Read the model definition and answer for the solid it produces. Units are mm, in the model's axes. A direction names the side the tool comes from. Give positions to 0.01 mm unless a question says otherwise; leave off trailing zeros. Loops run counter-clockwise (first coordinate to the right, second up) from the corner with the lowest first, then second, coordinate; pieces in that order, holes last. Notation, with made-up numbers: (57, 51.5) - (115, 51.5) arc R18 cw to (115, 69.5) - close; hole circle Ø9 at (-9, 38). An arc over 180 degrees is marked (long way). Write item = value, one per line.
```python
from build123d import *

# Parameters (mm, degrees)
F0_R      = 9.525
F1_DEPTH  = 15.8115
F2_R      = 11.1125
F3_DEPTH  = 7.112
F4_R      = 11.1125
F5_DEPTH  = 7.112
F6_T      = 3.175
F7_R      = 3.175
F8_DEPTH  = 3.175
F10_R     = 11.1125
F11_DEPTH = 1.5875


# Not quite as in the source:
# - a shell that OpenCascade refuses in one call is made with other operations: the cavity is built on its own and cut out


with BuildPart() as f1:
    # F0 (on Top) → F1 (new body)
    with BuildSketch(Plane.XY):
        with BuildLine():
            Line((-14.2875, 369.1638474552), (-14.2875, 0))
            ThreePointArc((-14.2875, 0), (-13.1999288208, -5.4675895399), (-10.1027881362, -10.1027881362))
            Line((-10.1027881362, -10.1027881362), (23.8125, -44.0180762724))
            Line((23.8125, -44.0180762724), (74.6125, -44.0180762724))
            Line((74.6125, -44.0180762724), (74.6125, 413.1819237276))
            Line((74.6125, 413.1819237276), (23.8125, 413.1819237276))
            Line((23.8125, 413.1819237276), (-10.1027881362, 379.2666355914))
            ThreePointArc((-10.1027881362, 379.2666355914), (-13.1999288208, 374.6314369951), (-14.2875, 369.1638474552))
        make_face()
        Circle(F0_R, mode=Mode.SUBTRACT)
        with Locations((0, 369.1638474552)):
            Circle(F0_R, mode=Mode.SUBTRACT)
    extrude(amount=F1_DEPTH)

    # F2 (on face) → F3 (cut)
    with BuildSketch(Plane.XY.offset(15.8115)):
        with Locations((0, 369.1638474552)):
            Circle(F2_R)
        Circle(F2_R)
    extrude(amount=-F3_DEPTH, mode=Mode.SUBTRACT)

    # F4 (on face) → F5 (cut)
    with BuildSketch(Plane(origin=(0, 0, 0), x_dir=(1, 0, 0), z_dir=(0, 0, -1))):
        Circle(F4_R)
        with Locations((0, -369.1638474552)):
            Circle(F4_R)
    extrude(amount=-F5_DEPTH, mode=Mode.SUBTRACT)

    # F6: shell of thickness 3.175, made by hand


with BuildPart() as f6_core1:
    # F6_t2: copy of F1
    add(f1.part)

    # the walls: a layer under each face that stays
    f6_faces = [f6_core1.faces().sort_by_distance(p)[0] for p in [
        (-13.1999288208, 374.6314369951, 7.90575),
        (6.8548559319, 396.2242796595, 7.90575),
        (-14.2875, 184.5819237276, 7.90575),
        (30.1625, 184.5819237276, 15.8115),
        (49.2125, 413.1819237276, 7.90575),
        (-13.1999288208, -5.4675895399, 7.90575),
        (74.6125, 184.5819237276, 7.90575),
        (6.8548559319, -27.0604322043, 7.90575),
        (49.2125, -44.0180762724, 7.90575),
        (-11.1125, 0, 3.556),
        (-11.1125, 369.1638474552, 3.556),
        (-11.1125, 0, 12.2555),
        (-11.1125, 369.1638474552, 12.2555),
        (-7.4083333333, 7.4083333333, 7.112),
        (-7.4083333333, 376.5721807885, 7.112),
        (-7.4083333333, -7.4083333333, 8.6995),
        (-7.4083333333, 361.7555141219, 8.6995),
        (-9.525, 0, 7.90575),
        (-9.525, 369.1638474552, 7.90575),
    ]]
    thicken(f6_faces, amount=-F6_T, mode=Mode.SUBTRACT)

    # F6_s3 → F6_t4 (revolve, cut)
    with BuildSketch(Plane.XZ):
        Polygon((11.08075, 7.08025), (14.2875, 7.112), (14.2875, 10.287), (11.1125, 10.287), align=None)
    revolve(axis=Axis((0, 0, 7.112), (0, 0, -1)), mode=Mode.SUBTRACT)

    # F6_s5 → F6_t6 (revolve, cut)
    with BuildSketch(Plane.XZ.offset(-369.1638474552)):
        Polygon((11.08075, 7.08025), (14.2875, 7.112), (14.2875, 10.287), (11.1125, 10.287), align=None)
    revolve(axis=Axis((0, 369.1638474552, 7.112), (0, 0, -1)), mode=Mode.SUBTRACT)

    # F6_s7 → F6_t8 (revolve, cut)
    with BuildSketch(Plane.XZ):
        Polygon((11.08075, 8.73125), (14.2875, 8.6995), (14.2875, 5.5245), (11.1125, 5.5245), align=None)
    revolve(axis=Axis((0, 0, 8.6995), (0, 0, 1)), mode=Mode.SUBTRACT)

    # F6_s9 → F6_t10 (revolve, cut)
    with BuildSketch(Plane.XZ.offset(-369.1638474552)):
        Polygon((11.08075, 8.73125), (14.2875, 8.6995), (14.2875, 5.5245), (11.1125, 5.5245), align=None)
    revolve(axis=Axis((0, 369.1638474552, 8.6995), (0, 0, 1)), mode=Mode.SUBTRACT)


with BuildPart() as f1_1:
    add(f1.part)

    # what is left inside the walls is the cavity
    f6_cavity = [f6_core1.part.solids().sort_by_distance(p)[0] for p in [
        (30.1625, 109.440257, 12.60475),
    ]]
    add(f6_cavity, mode=Mode.SUBTRACT)

    # F7
    f7_edges = [f1_1.edges().sort_by_distance(p)[0] for p in [
        (-1.507724, 383.371572, 6.31825),
        (-11.1125, 360.183591, 6.31825),
        (-11.1125, 8.980256, 6.31825),
        (-1.507724, -14.207724, 6.31825),
    ]]
    fillet(f7_edges, radius=F7_R)

    # F8 (cut, through all): a face of the model
    f8_faces = [f1_1.faces().sort_by_distance(p)[0] for p in [
        (32.2546535053, 184.5819237276, 12.6365),
    ]]
    extrude(f8_faces, amount=-F8_DEPTH, mode=Mode.SUBTRACT)

    # F10 (on offset) → F11 (join, symmetric)
    with BuildSketch(Plane.XY.offset(7.90575)):
        with BuildLine():
            Line((74.6125, -44.0180762724), (74.6125, 413.1819237276))
            Line((74.6125, 413.1819237276), (23.8125, 413.1819237276))
            Line((23.8125, 413.1819237276), (-10.1027881362, 379.2666355914))
            ThreePointArc((-10.1027881362, 379.2666355914), (-13.1999288208, 374.6314369951), (-14.2875, 369.1638474552))
            Line((-14.2875, 369.1638474552), (-14.2875, 0))
            ThreePointArc((-14.2875, 0), (-13.1999288208, -5.4675895399), (-10.1027881362, -10.1027881362))
            Line((-10.1027881362, -10.1027881362), (23.8125, -44.0180762724))
            Line((23.8125, -44.0180762724), (74.6125, -44.0180762724))
        make_face()
        Circle(F10_R, mode=Mode.SUBTRACT)
        with Locations((0, 369.1638474552)):
            Circle(F10_R, mode=Mode.SUBTRACT)
    extrude(amount=F11_DEPTH, both=True)


solid = f1_1.part
```
1) Each of these flat-tipped pins is pushed along its axis until it touches: P1, Ø6, axis at x = -3.5, z = 2, coming from the -Y side; P2, Ø6.5, axis at x = 5, y = 372.5, coming from the +Z side; P3, Ø5, axis at x = 5, z = 11.5, coming from the +Y side; P4, Ø1, axis at x = 9.5, y = 261.5, coming from the +Z side. Where does it stop, or does it pass through?
Output:
P1 = -19.71
P2 = through
P3 = 396.87
P4 = 9.49
2) A cutting plane is placed at A-A on x = 49.5. Determine the outline of the cut face in (y, z).
Output:
outline = (-44.02, 0) - (-40.84, 0) - (-40.84, 6.32) - (410.01, 6.32) - (410.01, 0) - (413.18, 0) - (413.18, 15.81) - (410.01, 15.81) - (410.01, 9.49) - (-40.84, 9.49) - (-40.84, 15.81) - (-44.02, 15.81) - close
3) The mould has two halves that part along X. Classify faces 4 (the face through (-13.23, -5.39, 7.8)), 5 (the face through (-5, -8.3, 7.112)), 6 (the face through (74.612, 181, 8)): pulls with the +X half, pulls with the -X half, needs draft (parallel to the pull), parting line crosses it, or undercut.
Output:
face_4 = pulls with the -X half
face_5 = undercut
face_6 = pulls with the +X half
4) Find the intervals of material crossed by probe 1 along X at (y, z) = (0, 5); probe 2 along Y at (x, z) = (31.5, 1.5); probe 3 along X at (y, z) = (203, 14), in increasing order.
Output:
probe_1 = -14.29 to -11.11, 11.11 to 14.29, 71.44 to 74.61
probe_2 = -44.02 to -40.84, 410.01 to 413.18
probe_3 = -14.29 to -11.11, 71.44 to 74.61
5) A cutting plane is placed at B-B on y = 168.5. Determine the outline of the cut face in (x, z).
Output:
outline = (-14.29, 0) - (-11.11, 0) - (-11.11, 6.32) - (71.44, 6.32) - (71.44, 0) - (74.61, 0) - (74.61, 15.81) - (71.44, 15.81) - (71.44, 9.49) - (-11.11, 9.49) - (-11.11, 15.81) - (-14.29, 15.81) - close
6) A tool of negligible diameter and unlimited length cuts with its end or side. For faces 1 (the face through (14.29, 399.17, 12.61)), 2 (the face through (13.07, 363.39, 3.2)), 3 (the face through (6.617, -26.823, 8.016)), from which of +Z, -Z, +X, -X, +Y, -Y can it reach the whole face along a straight path? Write none if from no direction.
Output:
face_1 = +Z
face_2 = -Z
face_3 = +Z, -Z, -X, -Y
7) A cutting plane is placed at C-C on z = 2.5. Give the number of separate pieces and of enclosed holes in the cut face, then the cut area to 3 significant figures.
Output:
separate_pieces = 1
enclosed_holes = 3
area = 3,680 mm²
